CAD build for the part. Positions are in the model's coordinates, mm. A direction names the side the tool comes from. Give positions to 0.01 mm unless a question says otherwise; leave off trailing zeros. Loops run counter-clockwise (first coordinate to the right, second up) from the corner with the lowest first, then second, coordinate; pieces in that order, holes last.
Item 1: Which spindle directions (+Z, -Z, +X, -X, +Y, -Y) get a long thin tool onto all of the face, cutting with end or side? Do faces 4 (the flat face through (13.2, 4.4, -9.3)), 5 (the flat face through (7, 91.44, 10.1)), 6 (the flat face through (-0.635, 4, 16)), 7 (the flat face through (-13, 8.89, -9)). Say none if no direction does.
Item 2: Saw through at A-A on z = 0. Give the cut face in (x, y) (3 decimals).
Item 3: Saw through at B-B on y = 84. Give the cut face in (x, z) (3 decimals).
Item 4: Drop flat-ended pins along their axis: P1, Ø6.5, axis at y = 6.5, z = 17, coming from the -X side; P2, Ø0.5, axis at x = 2, z = 16, coming from the +Y side; P3, Ø1.2, axis at y = 93, z = 14, coming from the +X side; P4, Ø3, axis at x = -11.5, y = 96, coming from the +Z side. Give the stop position or say it passes through.
Item 5: Saw through at C-C on y = 25.5. Give the cut face in (x, z) (3 decimals), plus the area to 3 significant figures.
Item 6: Mould opens along Z. For faces 1 (the flat face through (11.1, 0, 5.3)), 2 (the conical face through (-12.316, 86.487, 6.881)), 3 (the cylindrical face through (-3.62, 46.36, -11.51)) say: released by +Z, released by -Z, zero draft, split by the parting line, or undercut.
Item 7: Probe probe 1 along X at (y, z) = (22, 0) (3 decimals); probe 2 along Z at (x, y) = (-4.5, 47.5). List the from-to ranges inside material, lowest first.
Autodesk Inventor part; units mm, degrees
ref_plane "Work Plane1" through (0, 0, 0) normal (0, -1, 0) x (1, 0, 0)
ref_plane "YZ Plane" through (0, 0, 0) normal (1, 0, 0) x (0, 1, 0)
ref_plane "XZ Plane" through (0, 0, 0) normal (0, 1, 0) x (-1, 0, 0)
sketch "Sketch1" plane through (0, 0, 0) normal (1, 0, 0) x (0, 1, 0)
  line L0 (0, 0) -> (0, -12.065)
  line L1 (0, -12.065) -> (91.44, -12.065)
  line L2 (91.44, -13.335) -> (0, -13.335)
  line L3 (0, -13.335) -> (0, -12.065)
  line L4 (0, 0) -> (110.5631, 0)
  line L5 (116.84, 0) -> (116.84, -13.589)
  line L6 (116.84, -13.589) -> (91.44, -13.589)
  line L7 (116.84, -13.589) -> (142.24, -13.589) construction
  line L8 (109.5817, -14.859) -> (91.44, -14.859)
  line L9 (91.44, -14.859) -> (81.393, -13.335)
  line L10 (91.44, -13.589) -> (91.44, -12.065)
  line L11 (116.84, -13.589) -> (109.5817, -14.859)
  point P0 (73.3806, -13.335)
  dimension "d0" = 12.065
  dimension "d1" = 91.44
  dimension "d39" = 13.589
  dimension "d41" = 180
ref_plane "Work Plane1" through (0, 0, 0) normal (0, -1, 0) x (1, 0, 0)
sketch "Sketch2" plane through (0, 0, 0) normal (0, -1, 0) x (1, 0, 0)
  circle A0 centre (0, 0) radius 13.335
  line L0 (11.2178, -7.2099) -> (16.1473, -10.0559)
  line L1 (11.8528, -6.11) -> (16.7823, -8.9561)
  line L2 (0.635, 13.3199) -> (0.635, 19.012)
  line L3 (-0.635, 13.3199) -> (-0.635, 19.012)
  line L4 (-11.8528, -6.11) -> (-16.7823, -8.9561)
  line L5 (-11.2178, -7.2099) -> (-16.1473, -10.0559)
  line L6 (16.1473, -10.0559) -> (16.7823, -8.9561)
  line L7 (0.635, 19.012) -> (-0.635, 19.012)
  line L8 (-16.7823, -8.9561) -> (-16.1473, -10.0559)
  line L9 (-0.635, 19.012) -> (-2.2892, 13.137)
  circle A1 centre (0, 0) radius 13.335
  line L10 (0.635, 19.012) -> (2.2723, 13.14)
  line L11 (16.7823, -8.9561) -> (12.5157, -4.6021)
  line L12 (-16.1473, -10.0559) -> (-10.2434, -8.5379)
  line L13 (-16.7823, -8.9561) -> (-12.5157, -4.6021)
  line L14 (16.1473, -10.0559) -> (10.2434, -8.5379)
  dimension "d24" = 6.096
  dimension "d25" = 6.096
  dimension "d27" = 6.096
  dimension "d28" = 6.096
  dimension "d29" = 6.096
extrude "Extrusion1" add sketch "Sketch2" against normal blind 8.89 contours A0 L2 L10 | L11 L1 A0 | A0 L9 L3 | L0 L14 A0 | A0 L4 L13 | L12 L5 A0
extrude "Extrusion2" cut sketch "Sketch2" against normal blind 124.7775 contours A0 L3 L7 L2 | L1 L6 L0 A0 | A0 L5 L8 L4
revolve "Revolution2" add sketch "Sketch1" angle 360 about axis through (0, 0, 0) along (0, 1, 0)
extrude "Extrusion3" cut sketch "Sketch2" against normal blind 174.625 contours A0 L3 L7 L2 | L1 L6 L0 A0 | A0 L5 L8 L4
properties part number "Engine_Holder_Mk_III" material "ABS Plastic"
Results below:
1. face 4: -Z, -Y
1. face 5: +Y
1. face 6: +Z, +Y, -Y
1. face 7: -Z, -X
2. outline: (-14.859, 91.44) - (-13.335, 81.393) - (-13.335, 0) - (-12.065, 0) - (-12.065, 91.44) - (-13.589, 91.44) - (-13.589, 116.84) - (-14.859, 109.582) - close; (12.065, 0) - (13.335, 0) - (13.335, 81.393) - (14.859, 91.44) - (14.859, 109.582) - (13.589, 116.84) - (13.589, 91.44) - (12.065, 91.44) - close
3. outline: (-12.196, -6.308) - (-11.853, -6.11) arc R13.335 ccw to (-11.218, -7.21) - (-11.561, -7.408) arc R13.73 ccw to (11.561, -7.408) - (11.218, -7.21) arc R13.335 ccw to (11.853, -6.11) - (12.196, -6.308) arc R13.73 ccw to (0.635, 13.716) - (0.635, 13.32) arc R13.335 ccw to (-0.635, 13.32) - (-0.635, 13.716) arc R13.73 ccw to start; hole circle Ø24.13 at (0, 0)
4. P1: stops at x = -2.12
4. P2: passes through
4. P3: stops at x = 6.42
4. P4: stops at z = 10.99
5. outline: circle Ø26.67 at (0, 0); hole circle Ø24.13 at (0, 0)
5. area: 101 mm2
6. face 1: zero draft
6. face 2: split by the parting line
6. face 3: undercut
7. probe 1: x = -13.335 to -12.065, 12.065 to 13.335
7. probe 2: z = -12.55 to -11.19, 11.19 to 12.55
